Source: CAD feature listing. Evaluate the final solid. Frame: model axes, mm. A direction names the side the tool comes from. Round coordinates to 2 decimals unless told otherwise and drop trailing zeros. Order: outer loops, then holes, each group sorted by start corner. A loop starts at its lowest first (then second) coordinate and runs counter-clockwise, first axis right, second up. Notation, with made-up numbers: (50, 53.5) -> (66, 53.5) arc R27 cw to (66, 91.5) -> close; hole circle Ø11 at (9.5, 57.5). An arc over 180 degrees is marked (long way). Use a Markdown table: item, result. Add a question column.
Autodesk Inventor part; units mm, degrees
ref_plane "YZ Plane" through (0, 0, 0) normal (1, 0, 0) x (0, 1, 0)
ref_plane "XZ Plane" through (0, 0, 0) normal (0, 1, 0) x (-1, 0, 0)
ref_plane "XY Plane" through (0, 0, 0) normal (0, 0, 1) x (1, 0, 0)
sketch "Sketch1" plane through (0, 0, 0) normal (0, 1, 0) x (-1, 0, 0)
  line L0 (0, 0) -> (0, 1200)
  line L1 (0, 1200) -> (240, 1200)
  line L2 (370, 400) -> (570, 400)
  line L3 (240, 1200) -> (370, 400)
  line L4 (570, 400) -> (570, 250)
  line L5 (570, 250) -> (370, 250)
  line L6 (370, 0) -> (370, 250)
  line L7 (370, 0) -> (280, 0)
  line L8 (280, 0) -> (280, 90)
  line L9 (280, 90) -> (90, 90)
  line L10 (90, 90) -> (90, 0)
  line L11 (90, 0) -> (0, 0)
  dimension "d2" = 1200
  dimension "d4" = 200
  dimension "d8" = 370
  dimension "d9" = 150
  dimension "d10" = 250
  dimension "d11" = 90
  dimension "d12" = 90
  dimension "d13" = 190
  dimension "d14" = 240
extrude "Extrusion1" add sketch "Sketch1" along normal blind 20
sketch "Sketch2" plane through (0, 0, 0) normal (0, -1, 0) x (1, 0, 0)
  line L0 (0, 0) -> (0, 1200)
  line L1 (0, 1200) -> (-240, 1200)
  line L2 (-240, 1200) -> (-240, 400)
  line L3 (-370, 400) -> (-570, 400)
  line L4 (-570, 400) -> (-570, 0)
  line L5 (-570, 0) -> (0, 0)
sketch "Sketch3" plane through (0, 0, 0) normal (0, -1, 0) x (1, 0, 0)
  line L0 (0, 0) -> (0, 1200)
  line L1 (0, 1200) -> (-240, 1200)
  line L2 (-240, 1200) -> (-370, 400)
  line L3 (-370, 400) -> (-570, 400)
  line L4 (-570, 400) -> (-570, 250)
  line L5 (-570, 250) -> (-370, 250)
  line L6 (-370, 250) -> (-370, 0)
  line L7 (-370, 0) -> (-280, 0)
  line L8 (-280, 0) -> (-280, 90)
  line L9 (-280, 90) -> (-90, 90)
  line L10 (-90, 90) -> (-90, 0)
  line L11 (-90, 0) -> (0, 0)
sketch "Sketch5" plane through (0, 20, 0) normal (0, 1, 0) x (1, 0, 0)
  line L0 (-8, -1190) -> (0, -1190)
  line L1 (0, 0) -> (-8, 0)
  line L2 (-8, 0) -> (-8, -1190)
  line L3 (-8, -1190) -> (0, -1190)
  line L4 (0, -1190) -> (0, 0)
  dimension "d18" = 8
  dimension "d21" = 8
  dimension "d22" = 1190
extrude "Extrusion3" cut sketch "Sketch5" against normal blind 10
properties part number "seitenteil"
1) Reachability of faces 1 (the flat face through (-90, 10, 46)), 2 (the flat face through (-370, 10, 123)), 3 (the flat face through (-469, 10, 400)) from +Z, -Z, +X, -X, +Y, -Y: full face, straight path, thin tool, end or side. Return the list, or none.
2) Section D-D on z = 451.5. Output: boundary loops of the cut face in (x, y), then the cut area to 3 significant figures.
3) Line query: probe 1 along Z at (x, y) = (-524, 10.5); probe 2 along Z at (x, y) = (-214.5, 18.5); probe 3 along X at (y, z) = (13, 165.5). Output: solid intervals per line, ascending. Write a range as from..to.
4) Section A-A on y = 4.75. Output: boundary loops of the cut face in (x, z).
5) Draft query along X for faces 4 (the flat face through (-186, 10, 90)), 5 (the flat face through (-326, 10, 0)), 6 (the flat face through (0, 5, 592)). Return one class per face: pulls with the +X half, pulls with the -X half, needs draft (parallel to the pull), parting line crosses it, or undercut.
6) Section C-C on x = -471. Output: boundary loops of the cut face in (y, z), then the cut area to 3 significant figures.
7) First-contact query: pin 1 Ø3 at (x, y) = (-399, 8.5) entering from +Z; pin 2 Ø6.5 at (x, z) = (-4, 791) entering from +Y; pin 3 Ø1 at (y, z) = (12.5, 914.5) entering from +X. Flat tips, straight axial feed; report the tip coordinate or a pass-through.
8) Section B-B on z = 187. Output: boundary loops of the cut face in (x, y), then the cut area to 3 significant figures.
Conclusion:
| question | item | result |
|---|---|---|
| 1 | face 1 | -Z, +Y, -Y |
| 1 | face 2 | -Z, -X, +Y, -Y |
| 1 | face 3 | +Z, -X, +Y, -Y |
| 2 | outline | (-361.63, 0) -> (0, 0) -> (0, 10) -> (-8, 10) -> (-8, 20) -> (-361.63, 20) -> close |
| 2 | area | 7,150 mm^2 |
| 3 | probe 1 | z = 250..400 |
| 3 | probe 2 | z = 90..1200 |
| 3 | probe 3 | x = -370..-8 |
| 4 | outline | (-570, 250) -> (-370, 250) -> (-370, 0) -> (-280, 0) -> (-280, 90) -> (-90, 90) -> (-90, 0) -> (0, 0) -> (0, 1200) -> (-240, 1200) -> (-370, 400) -> (-570, 400) -> close |
| 5 | face 4 | undercut |
| 5 | face 5 | needs draft |
| 5 | face 6 | pulls with the +X half |
| 6 | outline | (0, 250) -> (20, 250) -> (20, 400) -> (0, 400) -> close |
| 6 | area | 3,000 mm^2 |
| 7 | pin 1 | stops at z = 400 |
| 7 | pin 2 | stops at y = 10 |
| 7 | pin 3 | stops at x = -8 |
| 8 | outline | (-370, 0) -> (0, 0) -> (0, 10) -> (-8, 10) -> (-8, 20) -> (-370, 20) -> close |
| 8 | area | 7,320 mm^2 |
